```python
from build123d import *

# Parameters (mm, degrees)
F1_DEPTH = 62.4507963657
F2_W     = 60.3333711624
F2_H     = 19.3066857755
F4_DEPTH = 51.1555597186
F5_DEPTH = 25.4
F6_T     = -2.54


with BuildPart() as f1:
    # F0 (on Top) → F1 (new body)
    with BuildSketch(Plane.XY):
        Polygon((-39.5169705153, 66.5083825588), (-64.0413761139, 65.3912201524), (-62.551535666, -54.3909370899), (25.0678188681, -54.3909370899), (60.5918616056, -27.2963196039), (60.5918616056, 48.5934764147), (-39.5946651697, 48.5934764147), align=None)
    extrude(amount=F1_DEPTH)

    # F2 (on Top) → F4 (join)
    with BuildSketch(Plane.XY):
        with Locations((-33.4883257747, 38.7507472187)):
            Rectangle(F2_W, F2_H)
    extrude(amount=F4_DEPTH)

    # F5 (add): a face of the model
    f5_faces = [f1.faces().sort_by_distance(p)[0] for p in [
        (-4.8768218944, 0.8081448517, 62.4507963657),
    ]]
    extrude(f5_faces, amount=F5_DEPTH)

    # F6
    f6_openings = [f1.faces().sort_by_distance(p)[0] for p in [
        (-4.876822, 0.808145, 87.850796),
    ]]
    offset(amount=F6_T, openings=f6_openings, kind=Kind.INTERSECTION)


solid = f1.part
```
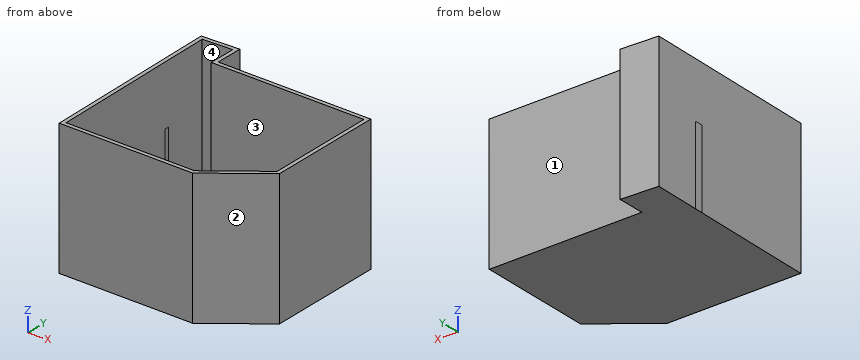
Geometry: final body of the model. Coordinates: model frame, mm. Face numbers are marked on the shaded views. Coordinates: 2 decimals unless noted, no trailing zeros. Order: outer loops, then holes, each group sorted by start corner. A loop starts at its lowest first (then second) coordinate and runs counter-clockwise, first axis right, second up. Notation, with made-up numbers: (3.5, 32) -> (48.5, 32) arc R26 cw to (48.5, 63) -> close; hole circle Ø2 at (4.25, 53.5). An arc over 180 degrees is marked (long way). Answer in a Markdown table with one row per item.
Item 1: Ray query, L1, parallel to Y at x = -38, z = 25; L2, parallel to Z at x = -43, y = 58; L3, parallel to X at y = -38, z = 23. Return the intervals inside material, ascending.
Return value:
| item | result |
|---|---|
| L1 | y = -54.39 to -51.85, 46.05 to 48.59 |
| L2 | z = 0 to 2.54 |
| L3 | x = -62.76 to -60.22, 42.37 to 46.56 |
Item 2: Section D-D on z = 81.5. Output: boundary loops of the cut face in (x, y), plus the area to 3 significant figures.
Return value:
| item | result |
|---|---|
| outline | (-64.04, 65.39) -> (-62.55, -54.39) -> (25.07, -54.39) -> (60.59, -27.3) -> (60.59, 48.59) -> (-39.59, 48.59) -> (-39.52, 66.51) -> close; hole (-61.47, 62.97) -> (-60.04, -51.85) -> (24.21, -51.85) -> (58.05, -26.04) -> (58.05, 46.05) -> (-42.15, 46.05) -> (-42.07, 63.85) -> close |
| area | 1,170 mm² |
Item 3: Section C-C on y = 55. Output: boundary loops of the cut face in (x, z).
Return value:
| item | result |
|---|---|
| outline | (-63.91, 0) -> (-39.57, 0) -> (-39.57, 87.85) -> (-42.11, 87.85) -> (-42.11, 2.54) -> (-61.37, 2.54) -> (-61.37, 87.85) -> (-63.91, 87.85) -> close |
Item 4: Contact query for flat-ended pins moving along their axis: P1, Ø10, axis at x = 22.5, z = 71, coming from the +Y side; P2, Ø1.6, axis at y = 31.5, z = 25, coming from the -X side (3 decimals); P3, Ø6, axis at x = 43, y = -10, coming from the +Z side; P4, Ø3, axis at x = -27, y = -1.5, coming from the -Z side. Output: stop coordinate, or through.
Return value:
| item | result |
|---|---|
| P1 | stops at y = 48.59 |
| P2 | stops at x = -63.655 |
| P3 | stops at z = 2.54 |
| P4 | stops at z = 0 |
Item 5: Section A-A on x = -33.5. Output: boundary loops of the cut face in (y, z), plus the area to 3 significant figures.
Return value:
| item | result |
|---|---|
| outline | (-54.39, 0) -> (48.59, 0) -> (48.59, 87.85) -> (46.05, 87.85) -> (46.05, 2.54) -> (-51.85, 2.54) -> (-51.85, 87.85) -> (-54.39, 87.85) -> close |
| area | 695 mm² |
Item 6: Draft query along Y for the marked faces 1, 2, 3 and 4. Return one class per face: released by +Y, released by -Y, zero draft, split by the parting line, or undercut.
Return value:
| item | result |
|---|---|
| face 1 | released by +Y |
| face 2 | released by -Y |
| face 3 | undercut |
| face 4 | undercut |
